Model file for the job. Use its own axes, mm. A direction names the side the tool comes from. Give positions to 0.01 mm unless a question says otherwise; leave off trailing zeros. Write each loop counter-clockwise with the first axis right and the second up, starting at its lowest first coordinate (ties: lowest second). Pieces come first, ordered by that corner, then holes. Notation, with made-up numbers: (42, 15.25) - (67, 15.25) arc R25 ccw to (67, 42.25) - close; hole circle Ø5 at (-2.75, 25.5). An arc over 180 degrees is marked (long way). One line per item, written item: value. Start each with the question number.
(1) Cut at A-A, the plane x = 0. List the corners of the cut face in (y, z), and give its area (3 significant figures).
(2) Cut at B-B, the plane y = -36. List the corners of the cut face in (x, z).
(3) Probe L1, parallel to X at y = -29.5, z = 21; L2, parallel to Y at x = -17.5, z = 39; L3, parallel to X at y = 49, z = 57. List the from-to ranges inside material, lowest first.
(4) Drop a flat-ended pin along its axis: P1, Ø4, axis at x = -17, z = 14, coming from the -Y side. Give the stop position or say it passes through.
(5) 3-axis set-ups, long thin cutter, end or side, ignore diameter. For faces 1 (the face through (-15, -7, 25)), 2 (the face through (17, -55.049, 12)), 3 (the face through (-17, -54.63, 12)), 4 (the face through (0, 19, 0)), 5 (the face through (13, -27, 12)): which of +Z, -Z, +X, -X, +Y, -Y reach the whole face in a straight line?
(6) Cut at D-D, the plane y = 17. List the corners of the cut face in (x, z), and give its area (3 significant figures).
(7) Cut at C-C, the plane z = 38. List the corners of the cut face in (x, y).
(8) Mould opens along Z. For faces 6 (the face through (-21.464, 17, 20)), 7 (the face through (0, 44, 75)), 8 (the face through (3.008, 43.733, 32.062)) say: pulls with the +Z half, pulls with the -Z half, needs draft (parallel to the pull), parting line crosses it, or undercut.
from build123d import *

# Parameters (mm, degrees)
F1_DEPTH = 25
F2_W     = 43.2835130529
F2_H     = 42.5491245473
F3_DEPTH = 50
F4_R     = 13.8760258661
F5_DEPTH = 119.7601809589


with BuildPart() as f1:
    # F0 (on Top) → F1 (new body)
    with BuildSketch(Plane.XY):
        with BuildLine():
            ThreePointArc((21.4635129483, 0), (19.2315893312, -9.5303913811), (13, -17.0787115463))
            Line((13, -17.0787115463), (13, -55.0494629913))
            Line((13, -55.0494629913), (21.8200001046, -55.0494629913))
            Line((21.8200001046, -55.0494629913), (21.8200001046, 0))
            Line((21.8200001046, 0), (21.8200001046, 64.7097179676))
            Line((21.8200001046, 64.7097179676), (-21.4635129483, 64.7097179676))
            Line((-21.4635129483, 64.7097179676), (-21.4635129483, 0))
            ThreePointArc((-21.4635129483, 0), (0, 21.4635129483), (21.4635129483, 0))
        make_face()
        with BuildLine():
            Line((-13, -54.6302845692), (-13, -17.0787115463))
            ThreePointArc((-13, -17.0787115463), (-19.2315893312, -9.5303913811), (-21.4635129483, 0))
            Line((-21.4635129483, 0), (-21.4635129483, -54.6302845692))
            Line((-21.4635129483, -54.6302845692), (-13, -54.6302845692))
        make_face()
        with BuildLine():
            ThreePointArc((-13, 0), (0, 13), (13, 0))
            Line((13, 0), (13, -17.0787115463))
            ThreePointArc((13, -17.0787115463), (19.2315893312, -9.5303913811), (21.4635129483, 0))
            ThreePointArc((21.4635129483, 0), (0, 21.4635129483), (-21.4635129483, 0))
            ThreePointArc((-21.4635129483, 0), (-19.2315893312, -9.5303913811), (-13, -17.0787115463))
            Line((-13, -17.0787115463), (-13, 0))
        make_face()
    extrude(amount=F1_DEPTH)

    # F2 (on face) → F3 (join)
    with BuildSketch(Plane.XY.offset(25)):
        with Locations((0.1782435782, 43.4351556939)):
            Rectangle(F2_W, F2_H)
    extrude(amount=F3_DEPTH)

    # F4 (on face) → F5 (cut, through all)
    with BuildSketch(Plane(origin=(0, 64.7097179676, 0), x_dir=(-1, 0, 0), z_dir=(0, 1, 0))):
        with Locations((0, 45.6084646285)):
            Circle(F4_R)
    extrude(amount=-F5_DEPTH, mode=Mode.SUBTRACT)


solid = f1.part
Answers follow:
1. outline: (13, 0) - (64.71, 0) - (64.71, 31.73) - (22.16, 31.73) - (22.16, 25) - (13, 25) - close; (22.16, 59.48) - (64.71, 59.48) - (64.71, 75) - (22.16, 75) - close
1. area: 2,240 mm²
2. outline: (-21.46, 0) - (-13, 0) - (-13, 25) - (-21.46, 25) - close; (13, 0) - (21.82, 0) - (21.82, 25) - (13, 25) - close
3. L1: x = -21.46 to -13, 13 to 21.82
3. L2: y = 22.16 to 64.71
3. L3: x = -21.46 to -7.92, 7.92 to 21.82
4. P1: stops at y = -54.63
5. face 1: +Z, +X, -X, -Y
5. face 2: +Z, -Z, +X, -X, -Y
5. face 3: +Z, -Z, -X, -Y
5. face 4: -Z, +X, -X, +Y, -Y
5. face 5: +Z, -Z, -Y
6. outline: (-21.46, 0) - (21.82, 0) - (21.82, 25) - (-21.46, 25) - close
6. area: 1,080 mm²
7. outline: (-21.46, 22.16) - (-11.6, 22.16) - (-11.6, 64.71) - (-21.46, 64.71) - close; (11.6, 22.16) - (21.82, 22.16) - (21.82, 64.71) - (11.6, 64.71) - close
8. face 6: needs draft
8. face 7: pulls with the +Z half
8. face 8: undercut
